```python
from build123d import *

# Parameters (mm, degrees)
CYLINDER007_R     = 10
CYLINDER007_DEPTH = 10
CYLINDER006_R     = 2
CYLINDER006_DEPTH = 10
CYLINDER005_R     = 2
CYLINDER005_DEPTH = 10
CYLINDER004_R     = 2
CYLINDER004_DEPTH = 10
CYLINDER003_R     = 2
CYLINDER003_DEPTH = 10
BOX002_W          = 42
BOX002_H          = 42
BOX002_DEPTH      = 10
CYLINDER002_R     = 2
CYLINDER002_DEPTH = 10
CYLINDER001_R     = 2
CYLINDER001_DEPTH = 10
CYLINDER_R        = 2
CYLINDER_DEPTH    = 10
BOX001_W          = 60
BOX001_H          = 20
BOX001_DEPTH      = 10
BOX_W             = 60
BOX_H             = 70
BOX_DEPTH         = 10
FILLET_R          = 5
FILLET001_R       = 5
FILLET002_R       = 3


with BuildPart() as cylinder007:
    # Cylinder007 → Cylinder007 (new body)
    with BuildSketch(Plane(origin=(30, 45, -1), x_dir=(1, 0, 0), z_dir=(0, 0, 1))):
        Circle(CYLINDER007_R)
    extrude(amount=CYLINDER007_DEPTH)


with BuildPart() as cylinder006:
    # Cylinder006 → Cylinder006 (new body)
    with BuildSketch(Plane(origin=(45, 30, -1), x_dir=(1, 0, 0), z_dir=(0, 0, 1))):
        Circle(CYLINDER006_R)
    extrude(amount=CYLINDER006_DEPTH)


with BuildPart() as cylinder005:
    # Cylinder005 → Cylinder005 (new body)
    with BuildSketch(Plane(origin=(45, 60, -1), x_dir=(1, 0, 0), z_dir=(0, 0, 1))):
        Circle(CYLINDER005_R)
    extrude(amount=CYLINDER005_DEPTH)


with BuildPart() as cylinder004:
    # Cylinder004 → Cylinder004 (new body)
    with BuildSketch(Plane(origin=(15, 60, -1), x_dir=(1, 0, 0), z_dir=(0, 0, 1))):
        Circle(CYLINDER004_R)
    extrude(amount=CYLINDER004_DEPTH)


with BuildPart() as cylinder003:
    # Cylinder003 → Cylinder003 (new body)
    with BuildSketch(Plane(origin=(15, 30, -1), x_dir=(1, 0, 0), z_dir=(0, 0, 1))):
        Circle(CYLINDER003_R)
    extrude(amount=CYLINDER003_DEPTH)


with BuildPart() as cube002:
    # Box002 → Box002 (new body)
    with BuildSketch(Plane(origin=(9, 24, 2), x_dir=(1, 0, 0), z_dir=(0, 0, 1))):
        with Locations((21, 21)):
            Rectangle(BOX002_W, BOX002_H)
    extrude(amount=BOX002_DEPTH)


with BuildPart() as cylinder002:
    # Cylinder002 → Cylinder002 (new body)
    with BuildSketch(Plane(origin=(50, 10, -1), x_dir=(1, 0, 0), z_dir=(0, 0, 1))):
        Circle(CYLINDER002_R)
    extrude(amount=CYLINDER002_DEPTH)


with BuildPart() as cylinder001:
    # Cylinder001 → Cylinder001 (new body)
    with BuildSketch(Plane(origin=(30, 10, -1), x_dir=(1, 0, 0), z_dir=(0, 0, 1))):
        Circle(CYLINDER001_R)
    extrude(amount=CYLINDER001_DEPTH)


with BuildPart() as cylinder:
    # Cylinder → Cylinder (new body)
    with BuildSketch(Plane(origin=(10, 10, -1), x_dir=(1, 0, 0), z_dir=(0, 0, 1))):
        Circle(CYLINDER_R)
    extrude(amount=CYLINDER_DEPTH)


with BuildPart() as cube001:
    # Box001 → Box001 (new body)
    with BuildSketch(Plane.XY.offset(5)):
        with Locations((30, 10)):
            Rectangle(BOX001_W, BOX001_H)
    extrude(amount=BOX001_DEPTH)


with BuildPart() as obj1:
    # Box → Box (new body)
    with BuildSketch(Plane.XY):
        with Locations((30, 35)):
            Rectangle(BOX_W, BOX_H)
    extrude(amount=BOX_DEPTH)

    # Cut: cut Cube001
    add(cube001.part, mode=Mode.SUBTRACT)

    # Cut001: cut Cylinder
    add(cylinder.part, mode=Mode.SUBTRACT)

    # Cut002: cut Cylinder001
    add(cylinder001.part, mode=Mode.SUBTRACT)

    # Cut003: cut Cylinder002
    add(cylinder002.part, mode=Mode.SUBTRACT)

    # Cut004: cut Cube002
    add(cube002.part, mode=Mode.SUBTRACT)

    # Cut005: cut Cylinder003
    add(cylinder003.part, mode=Mode.SUBTRACT)

    # Cut006: cut Cylinder004
    add(cylinder004.part, mode=Mode.SUBTRACT)

    # Cut007: cut Cylinder005
    add(cylinder005.part, mode=Mode.SUBTRACT)

    # Cut008: cut Cylinder006
    add(cylinder006.part, mode=Mode.SUBTRACT)

    # Fillet
    fillet_edges = [obj1.edges().sort_by_distance(p)[0] for p in [
        (0, 70, 5),
    ]]
    fillet(fillet_edges, radius=FILLET_R)

    # Fillet001
    fillet001_edges = [obj1.edges().sort_by_distance(p)[0] for p in [
        (60, 70, 5),
    ]]
    fillet(fillet001_edges, radius=FILLET001_R)

    # Fillet002
    fillet002_edges = [obj1.edges().sort_by_distance(p)[0] for p in [
        (51, 24, 6),
        (9, 24, 6),
        (51, 66, 6),
        (9, 66, 6),
    ]]
    fillet(fillet002_edges, radius=FILLET002_R)

    # Cut009: cut Cylinder007
    add(cylinder007.part, mode=Mode.SUBTRACT)


solid = obj1.part
```
Geometry: final body of the model. Coordinates: model frame, mm. A direction names the side the tool comes from. Coordinates: 2 decimals unless noted, no trailing zeros. Order: outer loops, then holes, each group sorted by start corner. A loop starts at its lowest first (then second) coordinate and runs counter-clockwise, first axis right, second up. Notation, with made-up numbers: (-21, 45) -> (30, 45) arc R30 ccw to (30, 73) -> close; hole circle Ø8 at (33, 66). An arc over 180 degrees is marked (long way). Answer in a Markdown table with one row per item.
Item 1: Access query for faces 1 (the cylindrical face through (58, 69, 5)), 2 (the cylindrical face through (9.86, 24.9, 6.06)). Directions: +Z, -Z, +X, -X, +Y, -Y. A direction counts if a zero-diameter tool reaches every point of the face in a straight line with its end or side. Return the directions, or none.
Return value:
| item | result |
|---|---|
| face 1 | +Z, -Z, +X, +Y |
| face 2 | +Z |
Item 2: Contact query for flat-ended pins moving along their axis: P1, Ø3, axis at x = 33.5, y = 28.5, coming from the +Z side; P2, Ø2.5, axis at x = 23, z = 7.5, coming from the -Y side; P3, Ø6, axis at x = 16, y = 13.5, coming from the +Z side. Output: stop coordinate, or through.
Return value:
| item | result |
|---|---|
| P1 | stops at z = 2 |
| P2 | stops at y = 20 |
| P3 | stops at z = 5 |
Item 3: Section A-A on y = 37. Output: boundary loops of the cut face in (x, z).
Return value:
| item | result |
|---|---|
| outline | (0, 0) -> (24, 0) -> (24, 2) -> (9, 2) -> (9, 10) -> (0, 10) -> close; (36, 0) -> (60, 0) -> (60, 10) -> (51, 10) -> (51, 2) -> (36, 2) -> close |
Item 4: Section C-C on z = 7.5. Output: boundary loops of the cut face in (x, y), plus the area to 3 significant figures.
Return value:
| item | result |
|---|---|
| outline | (0, 20) -> (60, 20) -> (60, 65) arc R5 ccw to (55, 70) -> (5, 70) arc R5 ccw to (0, 65) -> close; hole (9, 27) arc R3 ccw to (12, 24) -> (48, 24) arc R3 ccw to (51, 27) -> (51, 63) arc R3 ccw to (48, 66) -> (12, 66) arc R3 ccw to (9, 63) -> close |
| area | 1,230 mm² |
Item 5: Draft query along X for faces 3 (the flat face through (29.6, 12.4, 5)), 4 (the flat face through (60, 39, 5)), 5 (the cylindrical face through (51.908, 10.601, 2.465)), 6 (the cylindrical face through (1, 68, 5)). Return one class per face: released by +X, released by -X, zero draft, split by the parting line, or undercut.
Return value:
| item | result |
|---|---|
| face 3 | zero draft |
| face 4 | released by +X |
| face 5 | undercut |
| face 6 | released by -X |
Item 6: Section B-B on y = 10. Output: boundary loops of the cut face in (x, z), plus the area to 3 significant figures.
Return value:
| item | result |
|---|---|
| outline | (0, 0) -> (8, 0) -> (8, 5) -> (0, 5) -> close; (12, 0) -> (28, 0) -> (28, 5) -> (12, 5) -> close; (32, 0) -> (48, 0) -> (48, 5) -> (32, 5) -> close; (52, 0) -> (60, 0) -> (60, 5) -> (52, 5) -> close |
| area | 240 mm² |
Item 7: Ray query, L1, parallel to Y at x = 30, z = 3.75; L2, parallel to X at y = 30, z = 0.8; L3, parallel to X at y = 10, z = 3.15. Return the intervals inside material, ascending.
Return value:
| item | result |
|---|---|
| L1 | y = 0 to 8, 12 to 24, 66 to 70 |
| L2 | x = 0 to 13, 17 to 43, 47 to 60 |
| L3 | x = 0 to 8, 12 to 28, 32 to 48, 52 to 60 |
Item 8: Section D-D on x = 30. Output: boundary loops of the cut face in (y, z).
Return value:
| item | result |
|---|---|
| outline | (0, 0) -> (8, 0) -> (8, 5) -> (0, 5) -> close; (12, 0) -> (35, 0) -> (35, 2) -> (24, 2) -> (24, 10) -> (20, 10) -> (20, 5) -> (12, 5) -> close; (55, 0) -> (70, 0) -> (70, 10) -> (66, 10) -> (66, 2) -> (55, 2) -> close |
